Print and shaded views of the part. All mm, measured from the part's lowest x, y and z. Give positions to 0.01 mm unless a question says otherwise; leave off trailing zeros. Order: outer loops, then holes, each group sorted by start corner. A loop starts at its lowest first (then second) coordinate and runs counter-clockwise, first axis right, second up. Notation, with made-up numbers: (-9.5, 39.5) - (-1.5, 39.5) arc R30 cw to (-1.5, 71.5) - close; hole circle Ø11 at (70.25, 53). An arc over 180 degrees is marked (long way). Answer in a Markdown table with one row per item.
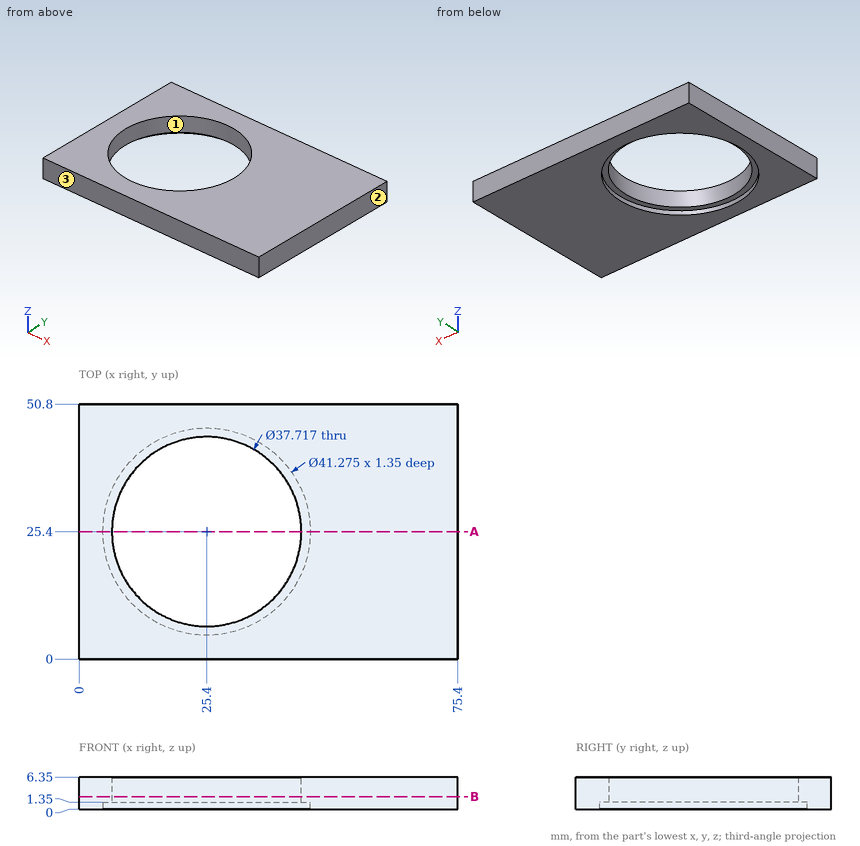
1. Two-plate mould, pull along X, no slides. Class the marked faces 1, 2 and 3: +X half, -X half, draft (parallel to the pull), parting line (faces both ways), or undercut.
Check result:
| item | result |
|---|---|
| face 1 | undercut |
| face 2 | +X half |
| face 3 | draft |
2. Cut at A-A on y = 25.4. Write the cut outline in (x, z).
Check result:
| item | result |
|---|---|
| outline | (0, 0) - (4.76, 0) - (4.76, 1.35) - (6.54, 1.35) - (6.54, 6.35) - (0, 6.35) - close; (44.26, 1.35) - (46.04, 1.35) - (46.04, 0) - (75.4, 0) - (75.4, 6.35) - (44.26, 6.35) - close |
3. Cut at B-B on z = 2.5. Write the cut outline in (x, y), and give its area (3 significant figures).
Check result:
| item | result |
|---|---|
| outline | (0, 0) - (75.4, 0) - (75.4, 50.8) - (0, 50.8) - close; hole circle Ø37.72 at (25.4, 25.4) |
| area | 2,710 mm² |
4. Probe line 1 (Y direction, x = 25.4, z = 0.7); line 2 (Y direction, x = 25.4, z = 3.1); line 3 (X direction, y = 15, z = 3.5). List the from-to ranges inside material, lowest first.
Check result:
| item | result |
|---|---|
| line 1 | y = 0 to 4.76, 46.04 to 50.8 |
| line 2 | y = 0 to 6.54, 44.26 to 50.8 |
| line 3 | x = 0 to 9.67, 41.13 to 75.4 |
